from build123d import *

# Parameters (mm, degrees)
BOSS_EXTRUDE1_DEPTH      = 4.35
BOSS_EXTRUDE1_DEPTH_BACK = 4.35
SKETCH3_R                = 2
BOSS_EXTRUDE2_DEPTH      = 111
SKETCH5_R                = 3.25
CUT_EXTRUDE1_DEPTH       = 113
CUT_EXTRUDE2_START       = -5
CUT_EXTRUDE2_DEPTH       = 6
SKETCH8_W                = 0.75
SKETCH8_H                = 4
BOSS_EXTRUDE4_DEPTH      = 3


with BuildPart() as part:
    # Sketch3 → Boss-Extrude1 (new, two sides: drawn at the far end of the back side and taken through both)
    with BuildSketch(Plane(origin=(0, 0, 0), x_dir=(1, 0, 0), z_dir=(0, 1, 0)).offset(-BOSS_EXTRUDE1_DEPTH_BACK)):
        with BuildLine():
            Line((0, 6), (-7, 6))
            Line((-7, 6), (-7, -6))
            Line((-7, -6), (0, -6))
            ThreePointArc((0, -6), (6, 0), (0, 6))
        make_face()
        with Locations(Location((0, 0, 0), (0, 0, 270))):
            Circle(SKETCH3_R, mode=Mode.SUBTRACT)
    extrude(amount=BOSS_EXTRUDE1_DEPTH + BOSS_EXTRUDE1_DEPTH_BACK)

    # Sketch4 → Boss-Extrude2 (add)
    with BuildSketch(Plane.ZY.offset(7)):
        Polygon((-6.375, -4.35), (6.375, -4.35), (6.375, 0.817855369), (6.375, 4.35), (-6.375, 4.35), (-6.375, -0.75), align=None)
    extrude(amount=BOSS_EXTRUDE2_DEPTH)

    # Sketch5 → Cut-Extrude1 (cut)
    with BuildSketch(Plane.ZY.offset(118)):
        Circle(SKETCH5_R)
    extrude(amount=-CUT_EXTRUDE1_DEPTH, mode=Mode.SUBTRACT)

    # Sketch6 → Cut-Extrude2 (cut)
    with BuildSketch(Plane.ZY.offset(118).offset(CUT_EXTRUDE2_START)):
        Polygon((-5.025, 0), (-5.025, 4.351777654), (-2.5125, 4.351777654), (2.5125, 4.351777654), (5.025, 4.351777654), (5.025, 0), (2.5125, -4.351777654), (-2.5125, -4.351777654), align=None)
    extrude(amount=-CUT_EXTRUDE2_DEPTH, mode=Mode.SUBTRACT)

    # Sketch8 → Boss-Extrude4 (add)
    with BuildSketch(Plane.ZY.offset(118)):
        with Locations((-6.75, 0)):
            Rectangle(SKETCH8_W, SKETCH8_H)
        with Locations((6.75, 0)):
            Rectangle(SKETCH8_W, SKETCH8_H)
    extrude(amount=-BOSS_EXTRUDE4_DEPTH)


solid = part.part
CAD build for the part. Positions are in the model's coordinates, mm. A direction names the side the tool comes from. Give positions to 0.01 mm unless a question says otherwise; leave off trailing zeros. Write each loop counter-clockwise with the first axis right and the second up, starting at its lowest first coordinate (ties: lowest second). Pieces come first, ordered by that corner, then holes. Notation, with made-up numbers: (36, -16) -> (58, -16) arc R20 cw to (58, 6) -> close; hole circle Ø2 at (-22, 75). An arc over 180 degrees is marked (long way). Return JSON: item names as keys, results as strings.
Item 1: Band-saw the part on B-B (x = -31.5). List the corners of the cut face in (y, z) (3 decimals).
Answer below:
{"outline": "(-4.35, -6.375) -> (4.35, -6.375) -> (4.35, 6.375) -> (-4.35, 6.375) -> close; hole circle Ø6.5 at (0, 0)"}
Item 2: Tool access for faces 1 (the cylindrical face through (-56.714, -1.978, -2.579)), 2 (the flat face through (-4, 0, 6)), 3 (the flat face through (-113, 3, -2)), 4 (the flat face through (-3, 0, -6)): list every direction of +Z, -Z, +X, -X, +Y, -Y with a clear straight run to the whole face (end or side of a thin tool).
Answer below:
{"face 1": "-X", "face 2": "+Z, +X, +Y, -Y", "face 3": "+Y", "face 4": "-Z, +X, +Y, -Y"}
Item 3: Two-plate mould, pull along X, no slides. Class faces 5 (the flat face through (-5, 0, 0)), 6 (the flat face through (-107, 3, -2)), 7 (the flat face through (-117, 0, 7.125)): +X half, -X half, draft (parallel to the pull), parting line (faces both ways), or undercut.
Answer below:
{"face 5": "-X half", "face 6": "undercut", "face 7": "draft"}
Item 4: Band-saw the part on A-A (z = 0). List the corners of the cut face in (x, y), then the cut area to 3 significant figures.
Answer below:
{"outline": "(-118, -4.35) -> (-113, -4.35) -> (-113, -3.25) -> (-118, -3.25) -> close; (-118, 3.25) -> (-113, 3.25) -> (-113, 4.35) -> (-118, 4.35) -> close; (-107, -4.35) -> (-2, -4.35) -> (-2, 4.35) -> (-107, 4.35) -> (-107, 3.25) -> (-5, 3.25) -> (-5, -3.25) -> (-107, -3.25) -> close; (2, -4.35) -> (6, -4.35) -> (6, 4.35) -> (2, 4.35) -> close", "area": "296 mm2"}
Item 5: Drill centre lines: probe 1 along Y at (x, z) = (-114.7, 0); probe 2 along X at (y, z) = (0.5, 0); probe 3 along X at (y, z) = (1.75, -1.5). Where is each one in solid material? Low to high.
Answer below:
{"probe 1": "y = -4.35 to -3.25, 3.25 to 4.35", "probe 2": "x = -5 to -2, 2 to 6", "probe 3": "x = -5 to -1.32, 1.32 to 5.81"}
Item 6: Drop flat-ended pins along their axis: pin 1 (4.5 mm diameter, centred on x = -39, y = -1, fed in from -Z) (3 decimals); pin 2 (0.6 mm diameter, centred on y = 0.5, z = -6.5, fed in from +X); pin 3 (0.8 mm diameter, centred on y = 0, z = 7, fed in from +X). Give the stop position or say it passes through.
Answer below:
{"pin 1": "stops at z = -6.375", "pin 2": "stops at x = -7", "pin 3": "stops at x = -115"}
